from build123d import *

# Parameters (mm, degrees)
SKETCH1_W           = 40
SKETCH1_H           = 36
BOSS_EXTRUDE1_DEPTH = 8
SKETCH2_R           = 5
CUT_EXTRUDE1_DEPTH  = 55.405882035
SKETCH3_W           = 20
SKETCH3_H           = 3.4
CUT_EXTRUDE2_DEPTH  = 55.405882035
SKETCH6_R           = 1.7
CUT_EXTRUDE3_DEPTH  = 55.405882035
SKETCH7_W           = 1
SKETCH7_H           = 7
CUT_EXTRUDE4_DEPTH  = 55.405882035


with BuildPart() as part:
    # Sketch1 → Boss-Extrude1 (new body)
    with BuildSketch(Plane(origin=(0, 0, 0), x_dir=(0, 0, -1), z_dir=(1, 0, 0))):
        with Locations((20, -18)):
            Rectangle(SKETCH1_W, SKETCH1_H)
    extrude(amount=BOSS_EXTRUDE1_DEPTH)

    # Sketch2 → Cut-Extrude1 (cut, through all)
    with BuildSketch(Plane(origin=(8, 0, 0), x_dir=(0, 0, -1), z_dir=(1, 0, 0))):
        with Locations((20, -18)):
            Circle(SKETCH2_R)
    extrude(amount=-CUT_EXTRUDE1_DEPTH, mode=Mode.SUBTRACT)

    # Sketch3 → Cut-Extrude2 (cut, through all)
    with BuildSketch(Plane(origin=(8, 0, 0), x_dir=(0, 0, -1), z_dir=(1, 0, 0))):
        with Locations((20, -5.5)):
            Rectangle(SKETCH3_W, SKETCH3_H)
        with Locations((20, -30.5)):
            Rectangle(SKETCH3_W, SKETCH3_H)
    extrude(amount=-CUT_EXTRUDE2_DEPTH, mode=Mode.SUBTRACT)

    # Sketch6 → Cut-Extrude3 (cut, through all)
    with BuildSketch(Plane(origin=(0, 0, 0), x_dir=(1, 0, 0), z_dir=(0, 1, 0))):
        with Locations(Location((4, 4, 0), (0, 0, 270))):
            Circle(SKETCH6_R)
        with Locations(Location((4, 36, 0), (0, 0, 270))):
            Circle(SKETCH6_R)
    extrude(amount=-CUT_EXTRUDE3_DEPTH, mode=Mode.SUBTRACT)

    # Sketch7 → Cut-Extrude4 (cut, through all)
    with BuildSketch(Plane(origin=(8, 0, 0), x_dir=(0, 0, -1), z_dir=(1, 0, 0))):
        with Locations((39.5, -7.5)):
            Rectangle(SKETCH7_W, SKETCH7_H)
    extrude(amount=-CUT_EXTRUDE4_DEPTH, mode=Mode.SUBTRACT)


solid = part.part
Input: part model. Units: mm. Frame: model coordinates. A direction names the side the tool comes from. Coordinates: 2 decimals unless noted, no trailing zeros. Loops run counter-clockwise (first coordinate to the right, second up) from the corner with the lowest first, then second, coordinate; pieces in that order, holes last. Notation, with made-up numbers: (20.5, -33) -> (75.5, -33) arc R18 ccw to (75.5, -12) -> close; hole circle Ø10 at (11.25, 41). An arc over 180 degrees is marked (long way). Write item = value, one per line. Start each with the question number.
Item 1: Cut plane C-C, the plane z = -20. Return loops of the section in (x, y).
Item 2: Cut plane D-D, the plane x = 1. Return loops of the section in (y, z).
Item 3: Reachability of faces 4 (the face through (4, -6, -10)), 5 (the face through (4, -8, -39)), 6 (the face through (8, -22, -24)) from +Z, -Z, +X, -X, +Y, -Y: full face, straight path, thin tool, end or side. Return the list, or none.
Item 4: First-contact query: P1, Ø1.7, axis at x = 3.5, y = -5, coming from the -Z side. Flat tip, straight axial feed; report the tip coordinate or a pass-through.
Item 5: Cut plane A-A, the plane x = 4. Return loops of the section in (y, z).
Item 6: Mould query, pull axis Z, two halves, no side actions, for faces 1 (the face through (4, -18, 0)), 2 (the face through (4, -31, -10)), 3 (the face through (4, -24, -40)). Classes: pulls with the +Z half, pulls with the -Z half, needs draft (parallel to the pull), parting line crosses it, or undercut.
Item 7: Material intervals for line 1 (Y direction, x = 7.75, z = -13); line 2 (X direction, y = -10.5, z = -4); line 3 (Z direction, x = 6.5, y = -31.5), sorted ascending.
Item 8: Cut plane B-B, the plane y = -5. Return loops of the section in (x, z).
Ans:
q1.outline = (0, -36) -> (8, -36) -> (8, -32.2) -> (0, -32.2) -> close; (0, -28.8) -> (8, -28.8) -> (8, -23) -> (0, -23) -> close; (0, -13) -> (8, -13) -> (8, -7.2) -> (0, -7.2) -> close; (0, -3.8) -> (8, -3.8) -> (8, 0) -> (0, 0) -> close
q2.outline = (-36, -40) -> (-11, -40) -> (-11, -39) -> (-4, -39) -> (-4, -40) -> (0, -40) -> (0, 0) -> (-36, 0) -> close; hole (-32.2, -30) -> (-28.8, -30) -> (-28.8, -10) -> (-32.2, -10) -> close; hole circle Ø10 at (-18, -20); hole (-7.2, -30) -> (-3.8, -30) -> (-3.8, -10) -> (-7.2, -10) -> close
q3.face_4 = +X, -X
q3.face_5 = -Z, +X, -X
q3.face_6 = +Z, -Z, +X, +Y, -Y
q4.P1 = -39
q5.outline = (-36, -40) -> (-11, -40) -> (-11, -39) -> (-4, -39) -> (-4, -40) -> (0, -40) -> (0, -37.7) -> (-36, -37.7) -> close; (-36, -34.3) -> (0, -34.3) -> (0, -5.7) -> (-36, -5.7) -> close; (-36, -2.3) -> (0, -2.3) -> (0, 0) -> (-36, 0) -> close; hole (-32.2, -30) -> (-28.8, -30) -> (-28.8, -10) -> (-32.2, -10) -> close; hole circle Ø10 at (-18, -20); hole (-7.2, -30) -> (-3.8, -30) -> (-3.8, -10) -> (-7.2, -10) -> close
q6.face_1 = pulls with the +Z half
q6.face_2 = undercut
q6.face_3 = pulls with the -Z half
q7.line_1 = -36 to -32.2, -28.8 to -7.2, -3.8 to 0
q7.line_2 = 0 to 2.3, 5.7 to 8
q7.line_3 = -40 to -30, -10 to 0
q8.outline = (0, -39) -> (8, -39) -> (8, -30) -> (0, -30) -> close; (0, -10) -> (8, -10) -> (8, 0) -> (0, 0) -> close; hole circle Ø3.4 at (4, -36); hole circle Ø3.4 at (4, -4)
